Geometry check sheet. Reference: the model listing, model coordinates, mm. Face numbers are marked on the shaded views. A direction names the side the tool comes from. Round coordinates to 2 decimals unless told otherwise and drop trailing zeros. Loops run counter-clockwise (first coordinate to the right, second up) from the corner with the lowest first, then second, coordinate; pieces in that order, holes last. Notation, with made-up numbers: M -1,-29 L 28,-29 A36 cw 28,5 Z; hole C 17.5,42 d5. An arc over 180 degrees is marked long. Use one line per item in the form item = value. Start each with the question number.
1. Set-up check for the marked faces 1, 2 and 3: record each of +Z, -Z, +X, -X, +Y, -Y from which the full face is reachable in a straight line by a thin tool's end or side.
2. Go/stop test with flat-tipped pins: pin 1 (2 mm diameter, centred on y = 57.5, z = 51.5, fed in from +X); pin 2 (6.5 mm diameter, centred on x = -61.78, z = -61.78, fed in from +Y); pin 3 (3 mm diameter, centred on x = 86.29, z = 13.67, fed in from -Y); pin 4 (5 mm diameter, centred on x = 39.66, z = 77.84, fed in from -Y). Record where each tip stops, or that it passes through.
3. Cross-section at B-B (y = 26). Record the boundary of the cut face in (x, z), then the cut area to 3 significant figures.
4. Cross-section at A-A (x = 9). Record the boundary of the cut face in (y, z), then the cut area to 3 significant figures.
5. Material ranges on line 1 (Z direction, x = -87, y = 15.5); line 2 (Y direction, x = -60, z = 66.5); line 3 (Z direction, x = 27, y = 12), recorded low to high.
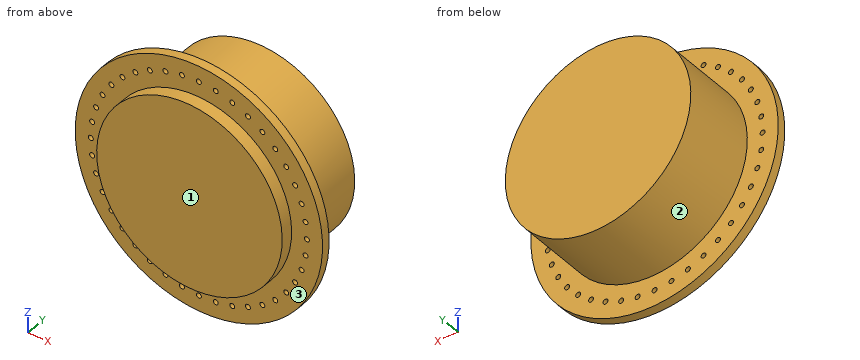
```python
from build123d import *

# Parameters (mm, degrees)
SKIZZE1_R                       = 75
AUFSATZ_LINEAR_AUSTRAGEN1_DEPTH = 10
SKIZZE2_R                       = 100
AUFSATZ_LINEAR_AUSTRAGEN2_DEPTH = 7
SKIZZE3_R                       = 75
AUFSATZ_LINEAR_AUSTRAGEN3_DEPTH = 60
SKIZZE4_R                       = 2
SCHNITT_LINEAR_AUSTRAGEN1_DEPTH = 60


with BuildPart() as part:
    # Skizze1 → Aufsatz-Linear austragen1 (new body)
    with BuildSketch(Plane(origin=(0, 0, 0), x_dir=(1, 0, 0), z_dir=(0, 1, 0))):
        with Locations(Location((0, 0, 0), (0, 0, 270))):
            Circle(SKIZZE1_R)
    extrude(amount=AUFSATZ_LINEAR_AUSTRAGEN1_DEPTH)

    # Skizze2 → Aufsatz-Linear austragen2 (add)
    with BuildSketch(Plane(origin=(0, 10, 0), x_dir=(1, 0, 0), z_dir=(0, 1, 0))):
        with Locations(Location((0, 0, 0), (0, 0, 270))):
            Circle(SKIZZE2_R)
    extrude(amount=AUFSATZ_LINEAR_AUSTRAGEN2_DEPTH)

    # Skizze3 → Aufsatz-Linear austragen3 (add)
    with BuildSketch(Plane(origin=(0, 17, 0), x_dir=(1, 0, 0), z_dir=(0, 1, 0))):
        with Locations(Location((0, 0, 0), (0, 0, 270))):
            Circle(SKIZZE3_R)
    extrude(amount=AUFSATZ_LINEAR_AUSTRAGEN3_DEPTH)

    # Skizze4 → Schnitt-Linear austragen1 (cut)
    with BuildSketch(Plane(origin=(0, 17, 0), x_dir=(1, 0, 0), z_dir=(0, 1, 0))):
        with Locations(Location((0, 87.36395499, 0), (0, 0, 270))):
            Circle(SKIZZE4_R)
        with Locations(Location((13.666733563, 86.288359732, 0), (0, 0, 270))):
            Circle(SKIZZE4_R)
        with Locations(Location((26.996946788, 83.088058682, 0), (0, 0, 270))):
            Circle(SKIZZE4_R)
        with Locations(Location((39.662405585, 77.841853875, 0), (0, 0, 270))):
            Circle(SKIZZE4_R)
        with Locations(Location((51.351244325, 70.678924283, 0), (0, 0, 270))):
            Circle(SKIZZE4_R)
        with Locations(Location((61.775645005, 61.775645005, 0), (0, 0, 270))):
            Circle(SKIZZE4_R)
        with Locations(Location((70.678924283, 51.351244325, 0), (0, 0, 270))):
            Circle(SKIZZE4_R)
        with Locations(Location((77.841853875, 39.662405585, 0), (0, 0, 270))):
            Circle(SKIZZE4_R)
        with Locations(Location((83.088058682, 26.996946788, 0), (0, 0, 270))):
            Circle(SKIZZE4_R)
        with Locations(Location((86.288359732, 13.666733563, 0), (0, 0, 270))):
            Circle(SKIZZE4_R)
        with Locations(Location((87.36395499, 0, 0), (0, 0, 270))):
            Circle(SKIZZE4_R)
        with Locations(Location((86.288359732, -13.666733563, 0), (0, 0, 270))):
            Circle(SKIZZE4_R)
        with Locations(Location((83.088058682, -26.996946788, 0), (0, 0, 270))):
            Circle(SKIZZE4_R)
        with Locations(Location((77.841853875, -39.662405585, 0), (0, 0, 270))):
            Circle(SKIZZE4_R)
        with Locations(Location((70.678924283, -51.351244325, 0), (0, 0, 270))):
            Circle(SKIZZE4_R)
        with Locations(Location((61.775645005, -61.775645005, 0), (0, 0, 270))):
            Circle(SKIZZE4_R)
        with Locations(Location((51.351244325, -70.678924283, 0), (0, 0, 270))):
            Circle(SKIZZE4_R)
        with Locations(Location((39.662405585, -77.841853875, 0), (0, 0, 270))):
            Circle(SKIZZE4_R)
        with Locations(Location((26.996946788, -83.088058682, 0), (0, 0, 270))):
            Circle(SKIZZE4_R)
        with Locations(Location((13.666733563, -86.288359732, 0), (0, 0, 270))):
            Circle(SKIZZE4_R)
        with Locations(Location((0, -87.36395499, 0), (0, 0, 270))):
            Circle(SKIZZE4_R)
        with Locations(Location((-13.666733563, -86.288359732, 0), (0, 0, 270))):
            Circle(SKIZZE4_R)
        with Locations(Location((-26.996946788, -83.088058682, 0), (0, 0, 270))):
            Circle(SKIZZE4_R)
        with Locations(Location((-39.662405585, -77.841853875, 0), (0, 0, 270))):
            Circle(SKIZZE4_R)
        with Locations(Location((-51.351244325, -70.678924283, 0), (0, 0, 270))):
            Circle(SKIZZE4_R)
        with Locations(Location((-61.775645005, -61.775645005, 0), (0, 0, 270))):
            Circle(SKIZZE4_R)
        with Locations(Location((-70.678924283, -51.351244325, 0), (0, 0, 270))):
            Circle(SKIZZE4_R)
        with Locations(Location((-77.841853875, -39.662405585, 0), (0, 0, 270))):
            Circle(SKIZZE4_R)
        with Locations(Location((-83.088058682, -26.996946788, 0), (0, 0, 270))):
            Circle(SKIZZE4_R)
        with Locations(Location((-86.288359732, -13.666733563, 0), (0, 0, 270))):
            Circle(SKIZZE4_R)
        with Locations(Location((-87.36395499, 0, 0), (0, 0, 270))):
            Circle(SKIZZE4_R)
        with Locations(Location((-86.288359732, 13.666733563, 0), (0, 0, 270))):
            Circle(SKIZZE4_R)
        with Locations(Location((-83.088058682, 26.996946788, 0), (0, 0, 270))):
            Circle(SKIZZE4_R)
        with Locations(Location((-77.841853875, 39.662405585, 0), (0, 0, 270))):
            Circle(SKIZZE4_R)
        with Locations(Location((-70.678924283, 51.351244325, 0), (0, 0, 270))):
            Circle(SKIZZE4_R)
        with Locations(Location((-61.775645005, 61.775645005, 0), (0, 0, 270))):
            Circle(SKIZZE4_R)
        with Locations(Location((-51.351244325, 70.678924283, 0), (0, 0, 270))):
            Circle(SKIZZE4_R)
        with Locations(Location((-39.662405585, 77.841853875, 0), (0, 0, 270))):
            Circle(SKIZZE4_R)
        with Locations(Location((-26.996946788, 83.088058682, 0), (0, 0, 270))):
            Circle(SKIZZE4_R)
        with Locations(Location((-13.666733563, 86.288359732, 0), (0, 0, 270))):
            Circle(SKIZZE4_R)
    extrude(amount=-SCHNITT_LINEAR_AUSTRAGEN1_DEPTH, mode=Mode.SUBTRACT)


solid = part.part
```
Reported:
q1.face_1 = +Z, -Z, +X, -X, -Y
q1.face_2 = +Y
q1.face_3 = -Y
q2.pin_1 = 55.45
q2.pin_2 = 17
q2.pin_3 = through
q2.pin_4 = 10
q3.outline = C 0,0 d150
q3.area = 17,700 mm²
q4.outline = M 0,-74.46 L 10,-74.46 L 10,-99.59 L 17,-99.59 L 17,-74.46 L 77,-74.46 L 77,74.46 L 17,74.46 L 17,99.59 L 10,99.59 L 10,74.46 L 0,74.46 Z
q4.area = 11,800 mm²
q5.line_1 = -49.31 to -15.54, -11.8 to -1.97, 1.97 to 11.8, 15.54 to 49.31
q5.line_2 = 10 to 17
q5.line_3 = -96.29 to -85.09, -81.09 to 81.09, 85.09 to 96.29
